from build123d import *

# Parameters (mm, degrees)
PAD_DEPTH       = 12
SKETCH001_R     = 4.8
POCKET_DEPTH    = 13
SKETCH006_W     = 12
SKETCH006_H     = 32
PAD001_DEPTH    = 15
SKETCH007_W     = 24
SKETCH007_H     = 12.5
POCKET004_DEPTH = 13
SKETCH008_R     = 3
POCKET005_DEPTH = 13
SKETCH009_W     = 11.997705
SKETCH009_H     = 19.984946
PAD002_DEPTH    = 12
FILLET_R        = 11
FILLET001_R     = 8


with BuildPart() as part:
    # Sketch → Pad (new body)
    with BuildSketch(Plane.XY):
        Polygon((0, 0), (23.300841, 0), (23.300841, 12), (-46.699159, 12), (-46.699159, -28), (-34.699159, -28), (-34.699159, 0), align=None)
    extrude(amount=PAD_DEPTH)

    # Sketch001 (on Face3 of Pad) → Pocket (cut)
    with BuildSketch(Plane(origin=(0, 12, 0), x_dir=(-1, 0, 0), z_dir=(0, 1, 0))):
        with Locations((-17, 6)):
            Circle(SKETCH001_R)
    extrude(amount=-POCKET_DEPTH, mode=Mode.SUBTRACT)

    # Sketch006 → Pad001 (join)
    with BuildSketch(Plane.XY.offset(12)):
        with Locations((4.232911, 16)):
            Rectangle(SKETCH006_W, SKETCH006_H)
    extrude(amount=PAD001_DEPTH)

    # Sketch007 (on Face19 of Pad001) → Pocket004 (cut)
    with BuildSketch(Plane.YZ.offset(10.232911)):
        with Locations((16.158846, 19.395833)):
            Rectangle(SKETCH007_W, SKETCH007_H)
    extrude(amount=-POCKET004_DEPTH, mode=Mode.SUBTRACT)

    # Sketch008 (on Face5 of Pocket004) → Pocket005 (cut)
    with BuildSketch(Plane(origin=(-46.699159, 0, 0), x_dir=(0, -1, 0), z_dir=(-1, 0, 0))):
        with Locations((16.234238, 6)):
            Circle(SKETCH008_R)
    extrude(amount=-POCKET005_DEPTH, mode=Mode.SUBTRACT)

    # Sketch009 (on Face12 of Pocket005) → Pad002 (join)
    with BuildSketch(Plane(origin=(0, 0, 12), x_dir=(1, 0, 0), z_dir=(0, 0, -1))):
        with Locations((4.247853, -21.997832)):
            Rectangle(SKETCH009_W, SKETCH009_H)
    extrude(amount=PAD002_DEPTH)

    # Fillet
    fillet_edges = [part.edges().sort_by_distance(p)[0] for p in [
        (4.247853, 31.990305, 0),
    ]]
    fillet(fillet_edges, radius=FILLET_R)

    # Fillet001
    fillet001_edges = [part.edges().sort_by_distance(p)[0] for p in [
        (-46.699159, 12, 6),
    ]]
    fillet(fillet001_edges, radius=FILLET001_R)


solid = part.part
Input: part model. Units: mm. Frame: model coordinates. A direction names the side the tool comes from. Coordinates: 2 decimals unless noted, no trailing zeros. Write each loop counter-clockwise with the first axis right and the second up, starting at its lowest first coordinate (ties: lowest second). Pieces come first, ordered by that corner, then holes. Notation, with made-up numbers: M 11,-6 L 27,-6 A14 ccw 27,14 Z; hole C 70,59 d7. An arc over 180 degrees is marked long. Answer as a JSON object with one key per item and string values. Group by question number.
(1) Mould query, pull axis Z, two halves, no side actions, for faces 4 (the face through (-7, 12, 6)), 5 (the face through (-20, 1, 0)), 6 (the face through (-46.699, -12, 6)). Classes: pulls with the +Z half, pulls with the -Z half, needs draft (parallel to the pull), parting line crosses it, or undercut.
(2) Set-up query: faces 1 (the face through (-6, 0, 10)), 2 (the face through (-30, 1, 12)), 3 (the face through (10.233, 16, 26)). Return all of +Z, -Z, +X, -X, +Y, -Y with unobstructed straight access to the full face (end or side cutting, diameter ignored); none if empty.
(3) Section A-A on x = 17. Output: boundary loops of the cut face in (y, z).
(4) Contact query for flat-ended pins moving along their axis: P1, Ø6, axis at y = -16.5, z = 7, coming from the +X side; P2, Ø3, axis at x = -19, y = -2, coming from the -Z side; P3, Ø9.5, axis at y = 26, z = 3.5, coming from the +X side; P4, Ø10, axis at x = -37.5, z = 15.5, coming from the +Y side. Output: stop coordinate, or through.
(5) Section B-B on z = 20.75. Output: boundary loops of the cut face in (x, y).
(6) Section D-D on z = 6. Output: boundary loops of the cut face in (x, y).
(7) Ray query, line 1 along Z through (x, y) = (17, 8.25); line 2 along Y through (x, z) = (-1.5, 14.25); line 3 along X through (y, z) = (-20.5, 9.5). Return the intervals inside material, ascending. Write a range as [from, to].
Result set:
{
 "1": {"face 4": "undercut", "face 5": "pulls with the -Z half", "face 6": "needs draft"},
 "2": {"face 1": "+Z, -Z, +X, -Y", "face 2": "+Z, -X, +Y, -Y", "face 3": "+Z, +X, +Y, -Y"},
 "3": {"outline": "M 0,0 L 12,0 L 12,1.2 L 0,1.2 Z; M 0,10.8 L 12,10.8 L 12,12 L 0,12 Z"},
 "4": {"P1": "stops at x = -34.7", "P2": "passes through", "P3": "stops at x = 10.25", "P4": "stops at y = 12"},
 "5": {"outline": "M -1.77,0 L 10.23,0 L 10.23,4.16 L -1.77,4.16 Z; M -1.77,28.16 L 10.23,28.16 L 10.23,32 L -1.77,32 Z"},
 "6": {"outline": "M -46.7,-28 L -34.7,-28 L -34.7,-19.23 L -46.7,-19.23 Z; M -46.7,-13.23 L -34.7,-13.23 L -34.7,0 L 12.2,0 L 12.2,12 L -38.7,12 A8 ccw -46.7,4 Z; M -1.75,12.01 L 10.25,12.01 L 10.25,30.79 L -1.75,30.79 Z; M 21.8,0 L 23.3,0 L 23.3,12 L 21.8,12 Z"},
 "7": {"line 1": "z = [0, 1.2], [10.8, 12]", "line 2": "y = [0, 4.16], [28.16, 32]", "line 3": "x = [-46.7, -34.7]"}
}
